Input: part model. Units: mm. Frame: model coordinates. Face numbers are marked on the shaded views. A direction names the side the tool comes from. Coordinates: 2 decimals unless noted, no trailing zeros. Loops run counter-clockwise (first coordinate to the right, second up) from the corner with the lowest first, then second, coordinate; pieces in that order, holes last.
(1) Contact query for flat-ended pins moving along their axis: P1, Ø3, axis at x = 10.5, z = -1.5, coming from the -Y side; P2, Ø1, axis at x = 19.5, y = 0, coming from the +Z side; P3, Ø1.5, axis at x = 15, z = 3, coming from the +Y side. Output: stop coordinate, or through.
(2) Set-up query: the marked faces 1, 2 and 3. Return all of +Z, -Z, +X, -X, +Y, -Y with unobstructed straight access to the full face (end or side cutting, diameter ignored); none if empty.
(3) Section B-B, the plane x = 28. Return loops of the section in (y, z), then the cut area to 3 significant figures.
(4) Line query: L1, parallel to X at y = 3.25, z = -0.75; L2, parallel to Z at x = 27.5, y = -2; L3, parallel to Y at x = 1, z = -1.5. Output: solid intervals per line, ascending.
(5) Mould query, pull axis X, two halves, no side actions, for the marked faces 4, 5 and 6. Classes: released by +X, released by -X, zero draft, split by the parting line, or undercut.
(6) Section C-C, the plane x = 18. Return loops of the section in (y, z).
(7) Section A-A, the plane z = 0. Return loops of the section in (x, y).
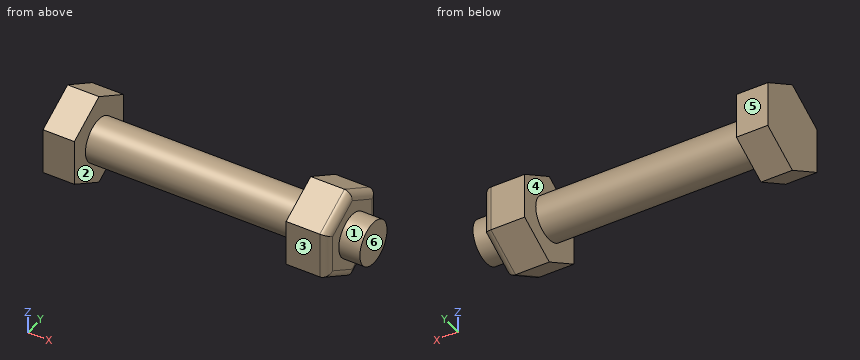
```python
from build123d import *

# Parameters (mm, degrees)
SKETCH1_W           = 35
SKETCH1_H           = 2.75
BOSS_EXTRUDE1_DEPTH = 4
BOSS_EXTRUDE2_DEPTH = 5.3
FILLET1_R           = 1


with BuildPart() as part:
    # Sketch1 → Revolve1 (revolve)
    with BuildSketch(Plane.XY):
        with Locations((17.5, 1.375)):
            Rectangle(SKETCH1_W, SKETCH1_H)
    revolve(axis=Axis((0, 0, 0), (1, 0, 0)))

    # Sketch2 → Boss-Extrude1 (add)
    with BuildSketch(Plane(origin=(0, 0, 0), x_dir=(0, 0, -1), z_dir=(1, 0, 0))):
        Polygon((5.773502692, 0), (2.886751346, 5), (-2.886751346, 5), (-5.773502692, 0), (-2.886751346, -5), (2.886751346, -5), align=None)
    extrude(amount=-BOSS_EXTRUDE1_DEPTH)

    # Sketch3 → Boss-Extrude2 (add)
    with BuildSketch(Plane(origin=(27, 0, 0), x_dir=(0, 0, -1), z_dir=(1, 0, 0))):
        Polygon((5.773502692, 0), (2.886751346, 5), (-2.886751346, 5), (-5.773502692, 0), (-2.886751346, -5), (2.886751346, -5), align=None)
    extrude(amount=BOSS_EXTRUDE2_DEPTH)

    # Fillet1
    fillet1_edges = [part.edges().sort_by_distance(p)[0] for p in [
        (32.3, -2.5, -4.330127019),
        (32.3, 2.5, -4.330127019),
        (32.3, 5, 0),
        (32.3, 2.5, 4.330127019),
        (32.3, -2.5, 4.330127019),
        (32.3, -5, 0),
    ]]
    fillet(fillet1_edges, radius=FILLET1_R)


solid = part.part
```
Report:
1. P1: stops at y = -2.75
1. P2: stops at z = 2.75
1. P3: stops at y = 1.58
2. face 1: +X
2. face 2: none
2. face 3: +Z, -Z, +X, -X, -Y
3. outline: (-5, -2.89) - (0, -5.77) - (5, -2.89) - (5, 2.89) - (0, 5.77) - (-5, 2.89) - close
3. area: 86.6 mm2
4. L1: x = -4 to 0, 27 to 32.3
4. L2: z = -4.62 to 4.62
4. L3: y = -2.3 to 2.3
5. face 4: undercut
5. face 5: zero draft
5. face 6: released by +X
6. outline: circle Ø5.5 at (0, 0)
7. outline: (-4, -5) - (0, -5) - (0, -2.75) - (27, -2.75) - (27, -5) - (31.3, -5) arc R1 ccw to (32.3, -4) - (32.3, -2.75) - (35, -2.75) - (35, 2.75) - (32.3, 2.75) - (32.3, 4) arc R1 ccw to (31.3, 5) - (27, 5) - (27, 2.75) - (0, 2.75) - (0, 5) - (-4, 5) - close
